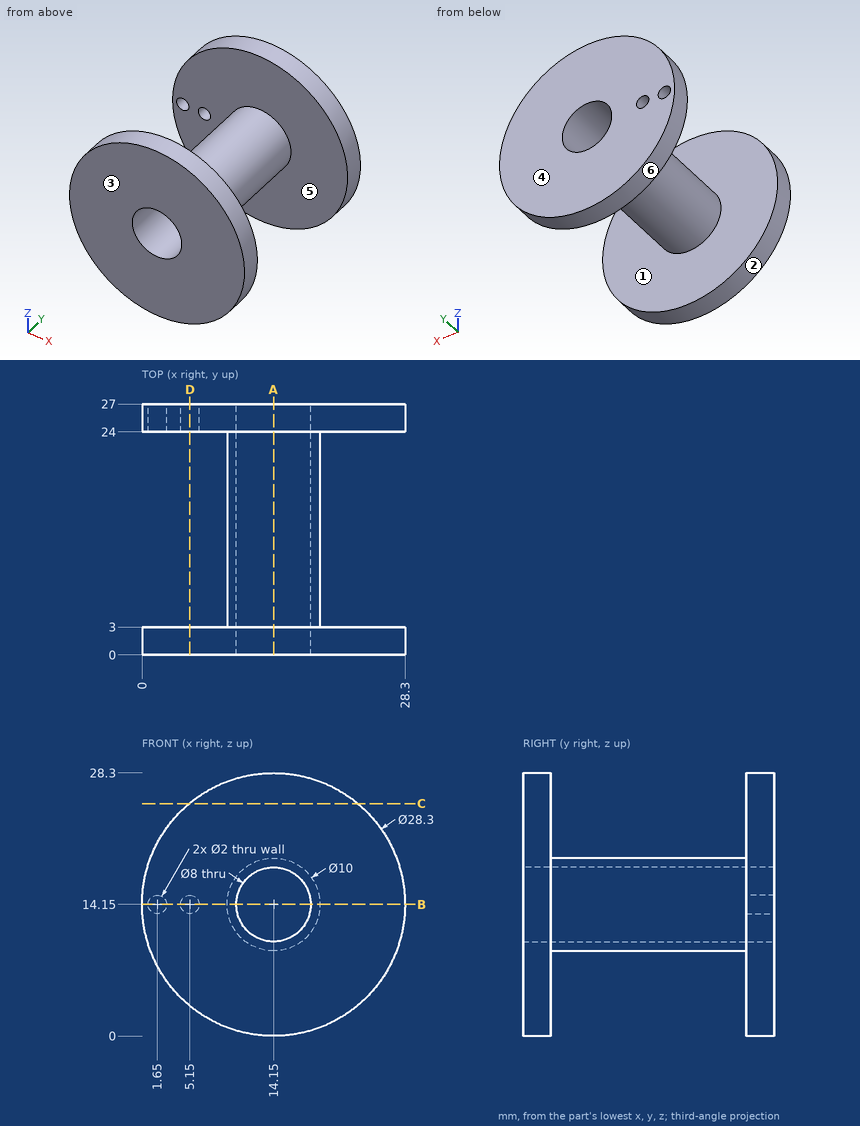
For this review, use the dimensioned drawing (mm, ordinates from the lowest corner) and the shaded views. A direction names the side the tool comes from. Give positions to 0.01 mm unless a question says otherwise; leave off trailing zeros. Write each loop counter-clockwise with the first axis right and the second up, starting at its lowest first coordinate (ties: lowest second). Pieces come first, ordered by that corner, then holes. Notation, with made-up numbers: M 66.5,75 L 75.5,75 A26 ccw 75.5,89 Z; hole C 4.25,-6 d6. An arc over 180 degrees is marked long. Write item = value, one per line. Start each with the question number.
Q1. Mouldability with a two-part tool opening along Y and no side actions: class the marked faces 3, 4, 5 and 6 as released by +Y, released by -Y, zero draft, split by the parting line, or undercut.
Q2. We need section A-A (x = 14.15). State the section outline as (y, z) points.
Q3. We need section B-B (z = 14.15). State the section outline as (x, y) points, plus the area to 3 significant figures.
Q4. For line 1 (X direction, y = 26.2, z = 14.15); line 2 (Y direction, x = 13.5, z = 2); line 3 (X direction, y = 14.5, z = 14.15), list the stretches that pass through material, from the lowest coordinate up.
Q5. Machinability: for the marked faces 1 and 2, which of the approach directions +Z, -Z, +X, -X, +Y, -Y give a long, thin tool a straight path to every point of the face, cutting with its end or side? Answer none if there is none.
Q6. We need section D-D (x = 5.15). State the section outline as (y, z) points, plus the area to 3 significant figures.
Q7. Clearance check with flat-ended pins moving along their axes: pin 1 (1.5 mm diameter, centred on y = 8, z = 20, fed in from +X); pin 2 (1 mm diameter, centred on x = 15.5, y = 18.5, fed in from -Z); pin 3 (3 mm diameter, centred on y = 9.5, z = 9, fed in from +X); pin 4 (12 mm diameter, centred on x = 22, y = 13.5, fed in from +Z). State where each tip first meets the part, or that it passes through.
Q8. We need section C-C (z = 25). State the section outline as (x, y) points.
Result set:
q1.face_3 = released by -Y
q1.face_4 = released by +Y
q1.face_5 = undercut
q1.face_6 = zero draft
q2.outline = M 0,0 L 3,0 L 3,9.15 L 24,9.15 L 24,0 L 27,0 L 27,10.15 L 0,10.15 Z; M 0,18.15 L 27,18.15 L 27,28.3 L 24,28.3 L 24,19.15 L 3,19.15 L 3,28.3 L 0,28.3 Z
q3.outline = M 0,0 L 10.15,0 L 10.15,27 L 6.15,27 L 6.15,24 L 9.15,24 L 9.15,3 L 0,3 Z; M 0,24 L 0.65,24 L 0.65,27 L 0,27 Z; M 2.65,24 L 4.15,24 L 4.15,27 L 2.65,27 Z; M 18.15,0 L 28.3,0 L 28.3,3 L 19.15,3 L 19.15,24 L 28.3,24 L 28.3,27 L 18.15,27 Z
q3.area = 152 mm2
q4.line_1 = 0 to 0.65, 2.65 to 4.15, 6.15 to 10.15, 18.15 to 28.3
q4.line_2 = 0 to 3, 24 to 27
q4.line_3 = 9.15 to 10.15, 18.15 to 19.15
q5.face_1 = none
q5.face_2 = +Y, -Y
q6.outline = M 0,3.23 L 3,3.23 L 3,25.07 L 0,25.07 Z; M 24,3.23 L 27,3.23 L 27,13.15 L 24,13.15 Z; M 24,15.15 L 27,15.15 L 27,25.07 L 24,25.07 Z
q6.area = 125 mm2
q7.pin_1 = through
q7.pin_2 = 9.22
q7.pin_3 = 17.57
q7.pin_4 = 18.8
q8.outline = M 5.07,0 L 23.23,0 L 23.23,3 L 5.07,3 Z; M 5.07,24 L 23.23,24 L 23.23,27 L 5.07,27 Z
